```python
from build123d import *

# Parameters (mm, degrees)
F0_W     = 196
F0_H     = 188
F0_R     = 2.6
F0_W_2   = 92
F0_H_2   = 16
F1_DEPTH = 4
F0_R_2   = 3.05
F2_DEPTH = 3


with BuildPart() as f1:
    # F0 (on Top) → F1 (new body)
    with BuildSketch(Plane.XY):
        with Locations((98, 94)):
            Rectangle(F0_W, F0_H)
        with Locations((10, 6)):
            Circle(F0_R, mode=Mode.SUBTRACT)
        with Locations((38, 6)):
            Circle(F0_R, mode=Mode.SUBTRACT)
        with Locations((10, 32)):
            Circle(F0_R, mode=Mode.SUBTRACT)
        with Locations((38, 32)):
            Circle(F0_R, mode=Mode.SUBTRACT)
        with Locations((98, 10)):
            Rectangle(F0_W_2, F0_H_2, mode=Mode.SUBTRACT)
        with Locations((10, 65)):
            Circle(F0_R, mode=Mode.SUBTRACT)
        with Locations((38, 65)):
            Circle(F0_R, mode=Mode.SUBTRACT)
        with Locations((10, 91)):
            Circle(F0_R, mode=Mode.SUBTRACT)
        with Locations((38, 91)):
            Circle(F0_R, mode=Mode.SUBTRACT)
        with Locations((80.5, 78)):
            Circle(F0_R, mode=Mode.SUBTRACT)
        with Locations((158, 6)):
            Circle(F0_R, mode=Mode.SUBTRACT)
        with Locations((186, 6)):
            Circle(F0_R, mode=Mode.SUBTRACT)
        with Locations((158, 32)):
            Circle(F0_R, mode=Mode.SUBTRACT)
        with Locations((186, 32)):
            Circle(F0_R, mode=Mode.SUBTRACT)
        with Locations((115.5, 78)):
            Circle(F0_R, mode=Mode.SUBTRACT)
        with Locations((158, 65)):
            Circle(F0_R, mode=Mode.SUBTRACT)
        with Locations((186, 65)):
            Circle(F0_R, mode=Mode.SUBTRACT)
        with Locations((158, 91)):
            Circle(F0_R, mode=Mode.SUBTRACT)
        with Locations((186, 91)):
            Circle(F0_R, mode=Mode.SUBTRACT)
        with Locations((80.5, 102)):
            Circle(F0_R, mode=Mode.SUBTRACT)
        with Locations((98, 140)):
            Rectangle(F0_W_2, F0_H_2, mode=Mode.SUBTRACT)
        with Locations((10, 156)):
            Circle(F0_R, mode=Mode.SUBTRACT)
        with Locations((38, 156)):
            Circle(F0_R, mode=Mode.SUBTRACT)
        with Locations((10, 182)):
            Circle(F0_R, mode=Mode.SUBTRACT)
        with Locations((38, 182)):
            Circle(F0_R, mode=Mode.SUBTRACT)
        with Locations((115.5, 102)):
            Circle(F0_R, mode=Mode.SUBTRACT)
        with Locations((158, 156)):
            Circle(F0_R, mode=Mode.SUBTRACT)
        with Locations((186, 156)):
            Circle(F0_R, mode=Mode.SUBTRACT)
        with Locations((158, 182)):
            Circle(F0_R, mode=Mode.SUBTRACT)
        with Locations((186, 182)):
            Circle(F0_R, mode=Mode.SUBTRACT)
    extrude(amount=F1_DEPTH)

    # F0 (on Top) → F2 (join)
    with BuildSketch(Plane.XY):
        with Locations((98, 140)):
            Rectangle(F0_W_2, F0_H_2)
        with Locations((59, 140)):
            Circle(F0_R_2, mode=Mode.SUBTRACT)
        with Locations((137, 140)):
            Circle(F0_R_2, mode=Mode.SUBTRACT)
        with Locations((98, 10)):
            Rectangle(F0_W_2, F0_H_2)
        with Locations((59, 10)):
            Circle(F0_R_2, mode=Mode.SUBTRACT)
        with Locations((137, 10)):
            Circle(F0_R_2, mode=Mode.SUBTRACT)
    extrude(amount=F2_DEPTH)


solid = f1.part
```
The listing builds one solid part. Answer for the finished solid, in the listing's coordinates (mm). Coordinates: 2 decimals unless noted, no trailing zeros. Write each loop counter-clockwise with the first axis right and the second up, starting at its lowest first coordinate (ties: lowest second). Pieces come first, ordered by that corner, then holes. Notation, with made-up numbers: (45, 67.5) - (87, 67.5) arc R17 ccw to (87, 95.5) - close; hole circle Ø8 at (-15, 21.25). An arc over 180 degrees is marked (long way). Return JSON: item names as keys, results as strings. Group by question number.
1. A cutting plane is placed at C-C, the plane x = 59. Determine the outline of the cut face in (y, z).
2. A cutting plane is placed at B-B, the plane x = 186. Determine the outline of the cut face in (y, z).
3. A cutting plane is placed at D-D, the plane y = 156. Determine the outline of the cut face in (x, z), plus the area to 3 significant figures.
4. Given pin 1 (4 mm diameter, centred on x = 158, y = 156, fed in from +Z); pin 2 (6 mm diameter, centred on x = 80.5, y = 142, fed in from +Z), each flat-ended and moving along its own axis, determine where each tip first touches the part or whether it passes through.
5. Straight lines are drawn through the part: L1, parallel to Y at x = 121, z = 3.6; L2, parallel to X at y = 156, z = 1. For each, find the intervals that lie inside material, in ascending order.
6. Determine the mould class of faces 1 (the cylindrical face through (9.662, 8.578, 1.972)), 2 (the flat face through (97, 140, 3)), 3 (the flat face through (97, 95, 0)) for opening direction X: released by +X, released by -X, zero draft, split by the parting line, or undercut.
7. A cutting plane is placed at A-A, the plane y = 102. Determine the outline of the cut face in (x, z), plus the area to 3 significant figures.
Ans:
{
 "1": {"outline": "(0, 0) - (6.95, 0) - (6.95, 3) - (2, 3) - (2, 4) - (0, 4) - close; (13.05, 0) - (136.95, 0) - (136.95, 3) - (132, 3) - (132, 4) - (18, 4) - (18, 3) - (13.05, 3) - close; (143.05, 0) - (188, 0) - (188, 4) - (148, 4) - (148, 3) - (143.05, 3) - close"},
 "2": {"outline": "(0, 0) - (3.4, 0) - (3.4, 4) - (0, 4) - close; (8.6, 0) - (29.4, 0) - (29.4, 4) - (8.6, 4) - close; (34.6, 0) - (62.4, 0) - (62.4, 4) - (34.6, 4) - close; (67.6, 0) - (88.4, 0) - (88.4, 4) - (67.6, 4) - close; (93.6, 0) - (153.4, 0) - (153.4, 4) - (93.6, 4) - close; (158.6, 0) - (179.4, 0) - (179.4, 4) - (158.6, 4) - close; (184.6, 0) - (188, 0) - (188, 4) - (184.6, 4) - close"},
 "3": {"outline": "(0, 0) - (7.4, 0) - (7.4, 4) - (0, 4) - close; (12.6, 0) - (35.4, 0) - (35.4, 4) - (12.6, 4) - close; (40.6, 0) - (155.4, 0) - (155.4, 4) - (40.6, 4) - close; (160.6, 0) - (183.4, 0) - (183.4, 4) - (160.6, 4) - close; (188.6, 0) - (196, 0) - (196, 4) - (188.6, 4) - close", "area": "701 mm²"},
 "4": {"pin 1": "through", "pin 2": "z = 3"},
 "5": {"L1": "0 to 2, 18 to 132, 148 to 188", "L2": "0 to 7.4, 12.6 to 35.4, 40.6 to 155.4, 160.6 to 183.4, 188.6 to 196"},
 "6": {"face 1": "undercut", "face 2": "undercut", "face 3": "zero draft"},
 "7": {"outline": "(0, 0) - (77.9, 0) - (77.9, 4) - (0, 4) - close; (83.1, 0) - (112.9, 0) - (112.9, 4) - (83.1, 4) - close; (118.1, 0) - (196, 0) - (196, 4) - (118.1, 4) - close", "area": "742 mm²"}
}
